Can you work these out from the model? Positions are in its coordinate system, mm. Coordinates: 2 decimals unless noted, no trailing zeros. Write each loop counter-clockwise with the first axis right and the second up, starting at its lowest first coordinate (ties: lowest second). Pieces come first, ordered by that corner, then holes.
```python
from build123d import *

# Parameters (mm, degrees)
SKETCH2_W           = 10
SKETCH2_H           = 10
BOSS_EXTRUDE1_DEPTH = 0.5
FILLET1_R           = 1
SKETCH3_R           = 2
CUT_EXTRUDE1_DEPTH  = 0.5


with BuildPart() as part:
    # Sketch2 → Boss-Extrude1 (new body)
    with BuildSketch(Plane(origin=(0, 0, 0), x_dir=(1, 0, 0), z_dir=(0, 1, 0))):
        Rectangle(SKETCH2_W, SKETCH2_H)
    extrude(amount=BOSS_EXTRUDE1_DEPTH)

    # Fillet1
    fillet1_edges = [part.edges().sort_by_distance(p)[0] for p in [
        (-5, 0.25, -5),
        (5, 0.25, -5),
        (5, 0.25, 5),
        (-5, 0.25, 5),
    ]]
    fillet(fillet1_edges, radius=FILLET1_R)

    # Sketch3 → Cut-Extrude1 (cut)
    with BuildSketch(Plane(origin=(0, 0.5, 0), x_dir=(1, 0, 0), z_dir=(0, 1, 0))):
        with Locations(Location((0, 0, 0), (0, 0, 270))):
            Circle(SKETCH3_R)
    extrude(amount=-CUT_EXTRUDE1_DEPTH, mode=Mode.SUBTRACT)


solid = part.part
```
1. If we section it at A-A, the plane y = 0.3: List the corners of the cut face in (x, z) for me, plus the area to 3 significant figures.
2. We'd pull the mould along X, two halves only. Please class faces 1 (the face through (4.699, 0.254, 4.715)), 2 (the face through (-4.715, 0.254, 4.699)), 3 (the face through (-1.952, 0.254, -0.434)): released by +X, released by -X, zero draft, split by the parting line, or undercut.
3. If we section it at C-C, the plane x = 1.5: List the corners of the cut face in (y, z) for me, plus the area to 3 significant figures.
4. I'm going to push flat-ended pins straight in: P1, Ø3, axis at x = 1, z = -0.5, coming from the +Y side; P2, Ø3, axis at x = 0, z = 0, coming from the -Y side. Where does each tip first touch, or does it pass through?
5. If I drill on L1, parallel to X at y = 0.25, z = 0; L2, parallel to Z at x = -0.25, y = 0.1; L3, parallel to Z at x = -0.5, y = 0.35, over which ranges is the centre line in solid material (lowest first)?
6. If we section it at B-B, the plane z = 0: List the corners of the cut face in (x, y) for me, plus the area to 3 significant figures.
Answers:
1. outline: (-5, -4) arc R1 ccw to (-4, -5) - (4, -5) arc R1 ccw to (5, -4) - (5, 4) arc R1 ccw to (4, 5) - (-4, 5) arc R1 ccw to (-5, 4) - close; hole circle Ø4 at (0, 0)
1. area: 86.6 mm2
2. face 1: released by +X
2. face 2: released by -X
2. face 3: undercut
3. outline: (0, -5) - (0.5, -5) - (0.5, -1.32) - (0, -1.32) - close; (0, 1.32) - (0.5, 1.32) - (0.5, 5) - (0, 5) - close
3. area: 3.68 mm2
4. P1: stops at y = 0.5
4. P2: passes through
5. L1: x = -5 to -2, 2 to 5
5. L2: z = -5 to -1.98, 1.98 to 5
5. L3: z = -5 to -1.94, 1.94 to 5
6. outline: (-5, 0) - (-2, 0) - (-2, 0.5) - (-5, 0.5) - close; (2, 0) - (5, 0) - (5, 0.5) - (2, 0.5) - close
6. area: 3.00 mm2
